Source: CAD feature listing. Evaluate the final solid. Frame: model axes, mm. A direction names the side the tool comes from. Round coordinates to 2 decimals unless told otherwise and drop trailing zeros. Order: outer loops, then holes, each group sorted by start corner. A loop starts at its lowest first (then second) coordinate and runs counter-clockwise, first axis right, second up. Notation, with made-up numbers: (-7.5, -26.75) -> (30.5, -26.75) arc R16 cw to (30.5, -4.75) -> close; hole circle Ø1 at (57.25, -20.5). An arc over 180 degrees is marked (long way). Answer as CSV lines item,"result". Start each with the question number.
(1) Section query A-A (y = 4.5). Output: boundary loops of the cut face in (x, z).
(2) Section query D-D (x = 27). Output: boundary loops of the cut face in (y, z).
(3) Set-up query: faces 1 (the flat face through (65, 30, -52)), 2 (the flat face through (33.1, 13.6, 11)), 3 (the cylindrical face through (34.25, 14.43, 9.57)). Return all of +Z, -Z, +X, -X, +Y, -Y with unobstructed straight access to the full face (end or side cutting, diameter ignored); none if empty.
(4) Section query B-B (z = 6). Output: boundary loops of the cut face in (x, y), plus the area to 3 significant figures.
(5) Contact query for flat-ended pins moving along their axis: P1, Ø4, axis at x = 52, z = 5.5, coming from the +Y side; P2, Ø1, axis at y = 39.5, z = -35, coming from the -X side; P3, Ø6.5, axis at x = 36, y = 46, coming from the -Z side; P4, Ø6.5, axis at x = 51.5, y = 42.5, coming from the +Z side. Output: stop coordinate, or through.
(6) Section query C-C (z = -33). Output: boundary loops of the cut face in (x, y), plus the area to 3 significant figures.
(7) Line query: line 1 along Y through (x, z) = (21.5, 2); line 2 along Z through (x, y) = (62.5, 7.5); line 3 along X through (y, z) = (57, -10.5). Output: solid intervals per line, ascending. Write a range as from..to.
(8) Pull-direction query (X, two-part tool) for faces 4 (the flat face through (28.174, 29.58, 8.07)), 5 (the flat face through (39, 30, 0)), 6 (the flat face through (38.14, 13.53, 10.99)); classes: +X half, -X half, draft (parallel to the pull), parting line (faces both ways), or undercut.
```python
from build123d import *

# Parameters (mm, degrees)
SKETCH_1_W          = 45.073019954
SKETCH_1_H          = 60
SKETCH_1_R          = 1.525
EXTRUDE_1_DEPTH     = 3
SKETCH_2_W          = 10
SKETCH_2_H          = 60
EXTRUDE_2_DEPTH     = 10
HOLE_WIZARD_1_D     = 8.3
EXTRUDE_3_DEPTH     = 60
CUT_EXTRUDE_1_DEPTH = 0.7
HOLE_WIZARD_2_D     = 3
HOLE_WIZARD_2_DEPTH = 5
SKETCH_10_W         = 3
SKETCH_10_H         = 52
SKETCH_10_H_2       = 3
SKETCH_10_W_2       = 4
EXTRUDE_4_DEPTH     = 60


with BuildPart() as part:
    # 草图1 → 凸台-拉伸1 (new body)
    with BuildSketch(Plane.XY):
        with Locations((37.463490023, 30)):
            Rectangle(SKETCH_1_W, SKETCH_1_H)
        with Locations((20.831064203, 4.5)):
            Circle(SKETCH_1_R, mode=Mode.SUBTRACT)
        with Locations((50.351484989, 4.5)):
            Circle(SKETCH_1_R, mode=Mode.SUBTRACT)
        with Locations((20.926980046, 55.5)):
            Circle(SKETCH_1_R, mode=Mode.SUBTRACT)
        with Locations((50.351484989, 55.5)):
            Circle(SKETCH_1_R, mode=Mode.SUBTRACT)
    extrude(amount=EXTRUDE_1_DEPTH)

    # 草图2 → 凸台-拉伸2 (add)
    with BuildSketch(Plane.XY.offset(3)):
        with Locations((35.639232517, 30)):
            Rectangle(SKETCH_2_W, SKETCH_2_H)
    extrude(amount=EXTRUDE_2_DEPTH)

    # 孔1 (through all)
    with Locations(Plane(origin=(0, 0, 0), x_dir=(-1, 0, 0), z_dir=(0, -1, 0))):
        with Locations((-35.639232517, -5)):
            Hole(HOLE_WIZARD_1_D / 2)

    # 草图5 → 凸台-拉伸3 (add)
    with BuildSketch(Plane.XZ):
        Polygon((30.639232517, 13), (25.639232517, 3), (30.639232517, 3), align=None)
        Polygon((40.639232517, 13), (45.639232517, 3), (40.639232517, 3), align=None)
    extrude(amount=-EXTRUDE_3_DEPTH)

    # 草图7 → 切除-拉伸1 (cut, symmetric)
    with BuildSketch(Plane.XY.offset(11)):
        Polygon((37.313548298, 12.1), (38.987864079, 15), (37.313548298, 17.9), (33.964916737, 17.9), (32.290600956, 15), (33.964916737, 12.1), align=None)
        Polygon((38.987864079, 45), (37.313548298, 47.9), (33.964916737, 47.9), (32.290600956, 45), (33.964916737, 42.1), (37.313548298, 42.1), align=None)
    extrude(amount=CUT_EXTRUDE_1_DEPTH, both=True, mode=Mode.SUBTRACT)

    # 孔2
    with Locations(Plane.XY.offset(13)):
        with Locations((35.639232517, 45), (35.639232517, 15)):
            Hole(HOLE_WIZARD_2_D / 2, depth=HOLE_WIZARD_2_DEPTH)

    # 草图10 → 凸台-拉伸4 (add)
    with BuildSketch(Plane(origin=(0, 60, 0), x_dir=(1, 0, 0), z_dir=(0, 1, 0))):
        with Locations((65.5, 26)):
            Rectangle(SKETCH_10_W, SKETCH_10_H)
        with Locations((65.5, -1.5)):
            Rectangle(SKETCH_10_W, SKETCH_10_H_2)
        with Locations((62, -1.5)):
            Rectangle(SKETCH_10_W_2, SKETCH_10_H_2)
    extrude(amount=-EXTRUDE_4_DEPTH)


solid = part.part
```
Answer block:
1,outline,"(14.93, 0) -> (19.31, 0) -> (19.31, 3) -> (14.93, 3) -> close; (22.36, 0) -> (48.83, 0) -> (48.83, 3) -> (45.64, 3) -> (40.64, 13) -> (30.64, 13) -> (25.64, 3) -> (22.36, 3) -> close; (51.88, 0) -> (64, 0) -> (64, -52) -> (67, -52) -> (67, 3) -> (51.88, 3) -> close; hole circle Ø8.3 at (35.64, 5)"
2,outline,"(0, 0) -> (60, 0) -> (60, 5.72) -> (0, 5.72) -> close"
3,face 1,"-Z, +X, -X, +Y, -Y"
3,face 2,"none"
3,face 3,"+Z"
4,outline,"(27.14, 0) -> (31.61, 0) -> (31.61, 60) -> (27.14, 60) -> close; (39.67, 0) -> (44.14, 0) -> (44.14, 60) -> (39.67, 60) -> close"
4,area,"537 mm2"
5,P1,"through"
5,P2,"x = 64"
5,P3,"z = 0"
5,P4,"z = 3"
6,outline,"(64, 0) -> (67, 0) -> (67, 60) -> (64, 60) -> close"
6,area,"180 mm2"
7,line 1,"0..3.13, 5.87..54.09, 56.91..60"
7,line 2,"0..3"
7,line 3,"64..67"
8,face 4,"-X half"
8,face 5,"draft"
8,face 6,"undercut"
